Read the model definition and answer for the solid it produces. Units are mm, in the model's axes. Face numbers are marked on the shaded views. A direction names the side the tool comes from. Coordinates: 2 decimals unless noted, no trailing zeros. Write each loop counter-clockwise with the first axis right and the second up, starting at its lowest first coordinate (ties: lowest second). Pieces come first, ordered by that corner, then holes.
(1) Given pin 1 (13 mm diameter, centred on x = -10, z = 16, fed in from -Y); pin 2 (9 mm diameter, centred on y = 4, z = 9.5, fed in from -X); pin 3 (5 mm diameter, centred on y = 15, z = 28.5, fed in from -X); pin 4 (6 mm diameter, centred on y = -13.5, z = 13, fed in from +X), each flat-ended and moving along its own axis, determine where each tip first touches the part or whether it passes through.
(2) The part is cut by section B-B, the plane z = 13.5. Determine the outline of the cut face in (x, y), and give its area (3 significant figures).
(3) The part is cut by section A-A, the plane x = 8. Determine the outline of the cut face in (y, z).
(4) The part is cut by section C-C, the plane y = -12. Determine the outline of the cut face in (x, z), and give its area (3 significant figures).
(5) Which of the six approach directions +Z, -Z, +X, -X, +Y, -Y give full straight-line access (tool end or side, diameter ignored) to the marked faces 5, 6 and 7?
(6) Determine the mould class of the marked faces 1, 2, 3 and 4 for opening direction Z: pulls with the +Z half, pulls with the -Z half, needs draft (parallel to the pull), parting line crosses it, or undercut.
(7) Straight lines are drawn through the part: line 1 along Y through (x, z) = (5.5, 30.5); line 2 along Z through (x, y) = (-10, -14); line 3 along X through (y, z) = (-3, 17.5). For each, find the intervals that lie inside material, in ascending order.
(8) The part is cut by section D-D, the plane z = 26.5. Determine the outline of the cut face in (x, y).
```python
from build123d import *

# Parameters (mm, degrees)
F1_DEPTH = 32
F2_R     = 8
F3_DEPTH = 99.3
F5_DEPTH = 32


with BuildPart() as f1:
    # F0 (on Top) → F1 (new body)
    with BuildSketch(Plane.XY):
        Polygon((26, 9), (26, 20), (-26, 20), (-26, 9), (15, 9), (15, -9), (-26, -9), (-26, -20), (26, -20), (26, -9), align=None)
    extrude(amount=F1_DEPTH)

    # F2 (on face) → F3 (cut)
    with BuildSketch(Plane.XZ.offset(20)):
        with BuildLine():
            ThreePointArc((-26, 16.000000143), (-21.3137084484, 27.3137085495), (-10, 32))
            Line((-10, 32), (-26, 32))
            Line((-26, 32), (-26, 16.000000143))
        make_face()
        with BuildLine():
            Line((-26, 0), (-10, 0))
            ThreePointArc((-10, 0), (-21.3137085495, 4.6862915516), (-26, 16.000000143))
            Line((-26, 16.000000143), (-26, 0))
        make_face()
        with Locations((-10, 16)):
            Circle(F2_R)
    extrude(amount=-F3_DEPTH, mode=Mode.SUBTRACT)

    # F4 (on face) → F5 (join)
    with BuildSketch(Plane.YZ.offset(26)):
        with BuildLine():
            ThreePointArc((9, 16), (6.3639610307, 22.3639610307), (0, 25))
            Line((0, 25), (0, 16))
            Line((0, 16), (9, 16))
        make_face()
        with BuildLine():
            Line((0, 16), (0, 25))
            ThreePointArc((0, 25), (-6.3639610307, 22.3639610307), (-9, 16))
            Line((-9, 16), (0, 16))
        make_face()
        with BuildLine():
            Line((9, 16), (0, 16))
            Line((0, 16), (0, 7))
            ThreePointArc((0, 7), (6.3639610307, 9.6360389693), (9, 16))
        make_face()
        with BuildLine():
            Line((0, 7), (0, 16))
            Line((0, 16), (-9, 16))
            ThreePointArc((-9, 16), (-6.3639610307, 9.6360389693), (0, 7))
        make_face()
    extrude(amount=F5_DEPTH)


solid = f1.part
```
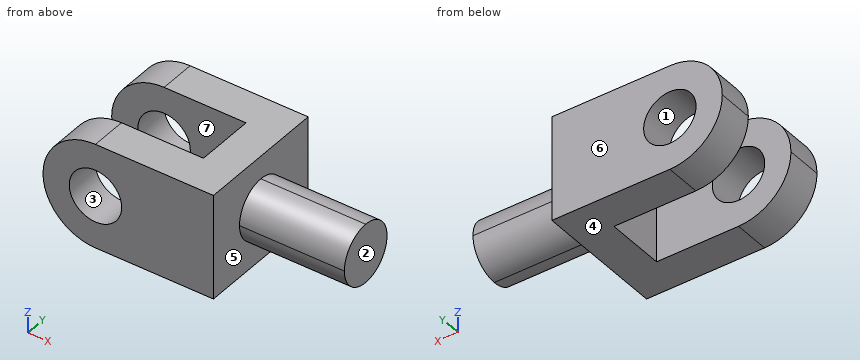
Computed:
1. pin 1: passes through
1. pin 2: stops at x = 15
1. pin 3: stops at x = -22.49
1. pin 4: stops at x = 26
2. outline: (-25.8, -20) - (-17.6, -20) - (-17.6, -9) - (-25.8, -9) - close; (-25.8, 9) - (-17.6, 9) - (-17.6, 20) - (-25.8, 20) - close; (-2.4, -20) - (26, -20) - (26, -8.65) - (58, -8.65) - (58, 8.65) - (26, 8.65) - (26, 20) - (-2.4, 20) - (-2.4, 9) - (15, 9) - (15, -9) - (-2.4, -9) - close
2. area: 1,560 mm2
3. outline: (-20, 0) - (-9, 0) - (-9, 32) - (-20, 32) - close; (9, 0) - (20, 0) - (20, 32) - (9, 32) - close
4. outline: (-10, 0) - (26, 0) - (26, 32) - (-10, 32) arc R16 ccw to start; hole circle Ø16 at (-10, 16)
4. area: 1,350 mm2
5. face 5: +X
5. face 6: +Z, -Z, +X, -X, +Y
5. face 7: +Z, -Z, -X
6. face 1: undercut
6. face 2: needs draft
6. face 3: undercut
6. face 4: pulls with the -Z half
7. line 1: y = -20 to -9, 9 to 20
7. line 2: z = 0 to 8, 24 to 32
7. line 3: x = 15 to 58
8. outline: (-22.07, -20) - (26, -20) - (26, 20) - (-22.07, 20) - (-22.07, 9) - (15, 9) - (15, -9) - (-22.07, -9) - close
